Read the model definition and answer for the solid it produces. Units are mm, in the model's axes. Face numbers are marked on the shaded views. A direction names the side the tool comes from. Coordinates: 2 decimals unless noted, no trailing zeros. Order: outer loops, then holes, each group sorted by start corner. A loop starts at its lowest first (then second) coordinate and runs counter-clockwise, first axis right, second up. Notation, with made-up numbers: (69, 36.25) - (120, 36.25) arc R23 cw to (120, 61.25) - close; hole circle Ø2 at (10.5, 17.25). An arc over 180 degrees is marked (long way). Use one line per item in the form item = value.
```python
from build123d import *

# Parameters (mm, degrees)
BASE_FLANGE1_DEPTH             = 0.8128
EDGE_FLANGE1_STRIP_W           = 6.4262
EDGE_FLANGE1_STRIP_H           = 0.8128
EDGE_FLANGE1_STRIP_CUT_DEPTH   = 35.042145822
EDGE_FLANGE1_STRIP_2_W         = 6.4262
EDGE_FLANGE1_STRIP_2_H         = 0.8128
EDGE_FLANGE1_STRIP_CUT_2_DEPTH = 35.042145822
EDGE_FLANGE1_DEPTH             = 35.042145822
EDGE_FLANGE1_BEND_DEPTH        = 35.042145822
SKETCH12_R                     = 6.35
CUT_EXTRUDE1_DEPTH             = 32.60643662
F_56_0_0465_DIAMETER_HOLE1_D   = 1.1811


# Sheet-metal steps are written as plain solids
with BuildPart() as part:
    # Sketch1 → Base-Flange1 (new body)
    with BuildSketch(Plane.XY):
        Polygon((-12.622145822, 8.32), (16.07, 8.32), (22.42, 8.32), (22.42, -8.27), (16.07, -8.27), (-12.622145822, -8.27), align=None)
    extrude(amount=BASE_FLANGE1_DEPTH)

    # Edge-Flange1 strip (across the edge) → Edge-Flange1 strip cut (cut)
    with BuildSketch(Plane(origin=(22.42, -8.27, 0), x_dir=(0, 1, 0), z_dir=(-1, 0, 0))):
        with Locations((-1.6256, -0.4064)):
            Rectangle(EDGE_FLANGE1_STRIP_W, EDGE_FLANGE1_STRIP_H)
    extrude(amount=EDGE_FLANGE1_STRIP_CUT_DEPTH, mode=Mode.SUBTRACT)

    # Edge-Flange1 strip 2 (across the edge) → Edge-Flange1 strip cut 2 (cut)
    with BuildSketch(Plane(origin=(-12.622145822, 8.32, 0), x_dir=(0, -1, 0), z_dir=(1, 0, 0))):
        with Locations((-1.6256, -0.4064)):
            Rectangle(EDGE_FLANGE1_STRIP_2_W, EDGE_FLANGE1_STRIP_2_H)
    extrude(amount=EDGE_FLANGE1_STRIP_CUT_2_DEPTH, mode=Mode.SUBTRACT)

    # Edge-Flange1 section (across the edge) → Edge-Flange1 (add)
    with BuildSketch(Plane(origin=(22.42, -8.27, 0), x_dir=(0, 1, 0), z_dir=(-1, 0, 0))):
        with BuildLine():
            Line((-0.8128, 1.5875), (-0.8128, 19.5072))
            Line((-0.8128, 19.5072), (0, 19.5072))
            Line((0, 19.5072), (0, 1.5875))
            ThreePointArc((0, 1.5875), (0.464967985, 0.464967985), (1.5875, 0))
            Line((1.5875, 0), (1.5875, -0.8128))
            ThreePointArc((1.5875, -0.8128), (-0.109768407, -0.109768407), (-0.8128, 1.5875))
        make_face()
    extrude(amount=EDGE_FLANGE1_DEPTH)

    # Edge-Flange1 section 2 (across the edge) → Edge-Flange1 bend (add)
    with BuildSketch(Plane(origin=(-12.622145822, 8.32, 0), x_dir=(0, -1, 0), z_dir=(1, 0, 0))):
        with BuildLine():
            Line((-0.8128, 1.5875), (-0.8128, 19.5072))
            Line((-0.8128, 19.5072), (0, 19.5072))
            Line((0, 19.5072), (0, 1.5875))
            ThreePointArc((0, 1.5875), (0.464967985, 0.464967985), (1.5875, 0))
            Line((1.5875, 0), (1.5875, -0.8128))
            ThreePointArc((1.5875, -0.8128), (-0.109768407, -0.109768407), (-0.8128, 1.5875))
        make_face()
    extrude(amount=EDGE_FLANGE1_BEND_DEPTH)

    # Sketch12 → Cut-Extrude1 (cut, through all)
    with BuildSketch(Plane.XY.offset(0.8128)):
        with Locations((2.127854178, 0.05)):
            Circle(SKETCH12_R)
    extrude(amount=-CUT_EXTRUDE1_DEPTH, mode=Mode.SUBTRACT)

    # #56 (0.0465) Diameter Hole1 (through all)
    with Locations(Plane(origin=(0, 9.1328, 0), x_dir=(1, 0, 0), z_dir=(0, 1, 0))):
        with Locations((19.245, 4.7625), (19.245, 16.3322), (-9.447145822, 16.3322), (-9.447145822, 4.7625)):
            Hole(F_56_0_0465_DIAMETER_HOLE1_D / 2)


solid = part.part
```
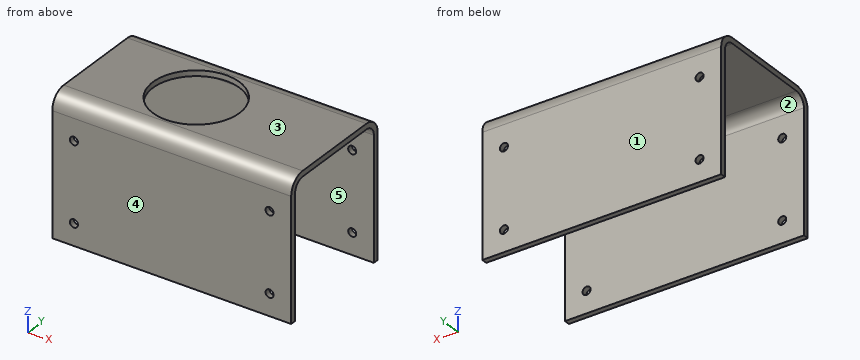
(1) Which of the six approach directions +Z, -Z, +X, -X, +Y, -Y give full straight-line access (tool end or side, diameter ignored) to the marked faces 1 and 2?
Answer list:
face_1 = +Z, -Z, +X, -X, +Y
face_2 = -Z, +X, -X
(2) Straight lines are drawn through the part: L1, parallel to Y at x = 0.5, z = -8; L2, parallel to Z at x = 13, y = 4.5; L3, parallel to Y at x = -0.5, z = 0.25. For each, find the intervals that lie inside material, in ascending order.
Answer list:
L1 = -9.08 to -8.27, 8.32 to 9.13
L2 = 0 to 0.81
L3 = -8.23 to -5.73, 5.83 to 8.28
(3) Section A-A, the plane z = -11.5 is taken. Write down the section's boundary in (x, y), then the cut area to 3 significant figures.
Answer list:
outline = (-12.62, -9.08) - (22.42, -9.08) - (22.42, -8.27) - (-12.62, -8.27) - close; (-12.62, 8.32) - (22.42, 8.32) - (22.42, 9.13) - (-12.62, 9.13) - close
area = 57.0 mm2
(4) Given pin 1 Ø1.5 at (x, y) = (18.5, 3) entering from -Z; pin 2 Ø10 at (y, z) = (-2, -6.5) entering from +X, each flat-ended and moving along its own axis, determine where each tip first touches the part or whether it passes through.
Answer list:
pin_1 = 0
pin_2 = through
(5) Section B-B, the plane y = -5.25 is taken. Write down the section's boundary in (x, z).
Answer list:
outline = (-12.62, 0) - (-1.37, 0) - (-1.37, 0.81) - (-12.62, 0.81) - close; (5.63, 0) - (22.42, 0) - (22.42, 0.81) - (5.63, 0.81) - close
(6) The mould has two halves that part along Y. Classify the marked faces 3, 4 and 5: +Y half, -Y half, draft (parallel to the pull), parting line (faces both ways), or undercut.
Answer list:
face_3 = draft
face_4 = -Y half
face_5 = undercut
